```python
from build123d import *

# Parameters (mm, degrees)
SKETCH2_W           = 35
SKETCH2_H           = 40
SKETCH2_R           = 1.75
BOSS_EXTRUDE2_DEPTH = 5.5
CUT_EXTRUDE1_REACH  = 10.5
CUT_EXTRUDE1_START  = -3
CUT_EXTRUDE2_START  = -3
CUT_EXTRUDE2_DEPTH  = 10
CUT_EXTRUDE3_DEPTH  = 6.5
FILLET3_R           = 5
FILLET4_R           = 8.5


with BuildPart() as part:
    # Sketch2 → Boss-Extrude2 (new body)
    with BuildSketch(Plane(origin=(0, 0, 0), x_dir=(1, 0, 0), z_dir=(0, 1, 0))):
        with Locations((17.5, 20)):
            Rectangle(SKETCH2_W, SKETCH2_H)
        with Locations((5, 35)):
            Circle(SKETCH2_R, mode=Mode.SUBTRACT)
        with Locations((30, 15)):
            Circle(SKETCH2_R, mode=Mode.SUBTRACT)
        with Locations((15, 35)):
            Circle(SKETCH2_R, mode=Mode.SUBTRACT)
        with Locations((15, 5)):
            Circle(SKETCH2_R, mode=Mode.SUBTRACT)
    extrude(amount=BOSS_EXTRUDE2_DEPTH)

    # Sketch3 → Cut-Extrude1 (cut, up to next)
    with BuildSketch(Plane.XZ.offset(CUT_EXTRUDE1_START), mode=Mode.PRIVATE) as cut_extrude1_sk1:
        Polygon((7.75, -36.58771324), (7.75, -33.41228676), (5, -31.824573519), (2.25, -33.41228676), (2.25, -36.58771324), (5, -38.175426481), align=None)
    cut_extrude1_tool1 = extrude(cut_extrude1_sk1.sketch, amount=-CUT_EXTRUDE1_REACH, mode=Mode.PRIVATE) & part.part
    add(cut_extrude1_tool1.solids().sort_by_distance((5, 3, -35))[0], mode=Mode.SUBTRACT)
    # Sketch3 → Cut-Extrude1 (cut, up to next)
    with BuildSketch(Plane.XZ.offset(CUT_EXTRUDE1_START), mode=Mode.PRIVATE) as cut_extrude1_sk2:
        Polygon((30, -11.824573519), (27.25, -13.41228676), (27.25, -16.58771324), (30, -18.175426481), (32.75, -16.58771324), (32.75, -13.41228676), align=None)
    cut_extrude1_tool2 = extrude(cut_extrude1_sk2.sketch, amount=-CUT_EXTRUDE1_REACH, mode=Mode.PRIVATE) & part.part
    add(cut_extrude1_tool2.solids().sort_by_distance((30, 3, -15))[0], mode=Mode.SUBTRACT)

    # Sketch4 → Cut-Extrude2 (cut)
    with BuildSketch(Plane(origin=(0, 5.5, 0), x_dir=(1, 0, 0), z_dir=(0, 1, 0)).offset(CUT_EXTRUDE2_START)):
        Polygon((17.75, 36.58771324), (15, 38.175426481), (12.25, 36.58771324), (12.25, 33.41228676), (15, 31.824573519), (17.75, 33.41228676), align=None)
        Polygon((13.41228676, 7.75), (11.824573519, 5), (13.41228676, 2.25), (16.58771324, 2.25), (18.175426481, 5), (16.58771324, 7.75), align=None)
    extrude(amount=-CUT_EXTRUDE2_DEPTH, mode=Mode.SUBTRACT)

    # Sketch5 → Cut-Extrude3 (cut, through all)
    with BuildSketch(Plane(origin=(0, 5.5, 0), x_dir=(1, 0, 0), z_dir=(0, 1, 0))):
        with BuildLine():
            Line((0, 36.58771324), (0, 40))
            Line((0, 40), (3.41228676, 40))
            ThreePointArc((3.41228676, 40), (0.999435653, 39.000564347), (0, 36.58771324))
        make_face()
        with BuildLine():
            Line((30, 19.75), (22, 19.75))
            Line((22, 19.75), (22, 40))
            Line((22, 40), (35, 40))
            Line((35, 40), (35, 0))
            Line((35, 0), (22, 0))
            Line((22, 0), (28, 10.25))
            Line((28, 10.25), (30, 10.25))
            ThreePointArc((30, 10.25), (34.75, 15), (30, 19.75))
        make_face()
        with BuildLine():
            Line((0, 34), (0, 0))
            Line((0, 0), (8, 0))
            Line((8, 0), (8, 29))
            Line((8, 29), (5, 29))
            ThreePointArc((5, 29), (1.464466094, 30.464466094), (0, 34))
        make_face()
    extrude(amount=-CUT_EXTRUDE3_DEPTH, mode=Mode.SUBTRACT)

    # Fillet3
    fillet3_edges = [part.edges().sort_by_distance(p)[0] for p in [
        (28, 2.75, -10.25),
        (22, 2.75, 0),
        (22, 2.75, -40),
        (8, 2.75, -29),
        (8, 2.75, 0),
    ]]
    fillet(fillet3_edges, radius=FILLET3_R)

    # Fillet4
    fillet4_edges = [part.edges().sort_by_distance(p)[0] for p in [
        (22, 2.75, -19.75),
    ]]
    fillet(fillet4_edges, radius=FILLET4_R)


solid = part.part
```
The model under review builds one solid part; all positions refer to its coordinate system, in mm. A direction names the side the tool comes from. Give positions to 0.01 mm unless a question says otherwise; leave off trailing zeros. Write each loop counter-clockwise with the first axis right and the second up, starting at its lowest first coordinate (ties: lowest second). Pieces come first, ordered by that corner, then holes. Notation, with made-up numbers: (57, 50) -> (100, 50) arc R24 cw to (100, 80) -> close; hole circle Ø9 at (67, -9.75). An arc over 180 degrees is marked (long way). Put each result on its own line as item: value.
(1) The part is to be moulded in two halves that separate along Z. For faces 4 (the cylindrical face through (20, 3, -39)), 5 (the flat face through (0, 3, -35)), 6 (the flat face through (12.63, 1.268, -6.394)), 7 (the flat face through (28.606, 4.232, -17.37)), say which applies: pulls with the +Z half, pulls with the -Z half, needs draft (parallel to the pull), parting line crosses it, or undercut.
Results are:
face 4: pulls with the -Z half
face 5: needs draft
face 6: undercut
face 7: undercut
(2) Tool access review of faces 1 (the flat face through (28.64, 4.23, -12.61)), 2 (the flat face through (16.36, 1.27, -32.61)), 3 (the cylindrical face through (1, 3, -31)): name each direction out of +Z, -Z, +X, -X, +Y, -Y from which nothing blocks a thin tool from reaching the whole face with its end or side.
Results are:
face 1: +Y
face 2: -Y
face 3: +Z, -X, +Y, -Y
(3) We need section C-C, the plane y = 3.9. State how many separate pieces and enclosed holes the cut face has, and give its area (3 significant figures).
Results are:
separate pieces: 1
enclosed holes: 4
area: 720 mm²
(4) For pin 1 Ø1.2 at (y, z) = (4.5, -35) entering from +X; pin 2 Ø1.6 at (x, z) = (15.5, -6) entering from -Y; pin 3 Ø2 at (x, y) = (20.5, 3) entering from +Z, all flat-tipped, find the tip position at first contact; note any pin that passes through.
Results are:
pin 1: x = 22
pin 2: y = 2.5
pin 3: z = -0.01
(5) We need section B-B, the plane z = -6. Give the boundary of the cut face in (x, y).
Results are:
outline: (8, 0) -> (12.4, 0) -> (12.4, 2.5) -> (13.56, 2.5) -> (13.56, 5.5) -> (8, 5.5) -> close; (16.44, 2.5) -> (17.6, 2.5) -> (17.6, 0) -> (25.51, 0) -> (25.51, 5.5) -> (16.44, 5.5) -> close
(6) We need section A-A, the plane z = -15. Give the boundary of the cut face in (x, y), and give its area (3 significant figures).
Results are:
outline: (8, 0) -> (28.25, 0) -> (28.25, 3) -> (27.25, 3) -> (27.25, 5.5) -> (8, 5.5) -> close; (31.75, 0) -> (34.75, 0) -> (34.75, 5.5) -> (32.75, 5.5) -> (32.75, 3) -> (31.75, 3) -> close
area: 123 mm²
(7) To check wall thickness, follow probe 1 along X at (y, z) = (2.2, -35); probe 2 along Z at (x, y) = (15, 4.65); probe 3 along X at (y, z) = (4.15, -35). State the ranges of each line that lie inside material, in increasing order. Write a range as from..to.
Results are:
probe 1: 0..3.25, 6.75..12.25, 17.75..22
probe 2: -40..-36.75, -33.25..-6.75, -3.25..0
probe 3: 0..2.25, 7.75..13.25, 16.75..22
